Build history of the part. All positions in model axes, mm. Face numbers are marked on the shaded views. A direction names the side the tool comes from. Round coordinates to 2 decimals unless told otherwise and drop trailing zeros. Write each loop counter-clockwise with the first axis right and the second up, starting at its lowest first coordinate (ties: lowest second). Pieces come first, ordered by that corner, then holes. Notation, with made-up numbers: M 4,-32.5 L 58,-32.5 A24 cw 58,-13.5 Z; hole C -39.5,26.25 d6. An arc over 180 degrees is marked long. Write item = value, one per line. Start each with the question number.
Q1. Tool access for the marked faces 4, 5, 6 and 7: list every direction of +Z, -Z, +X, -X, +Y, -Y with a clear straight run to the whole face (end or side of a thin tool).
Q2. Probe L1, parallel to Z at x = 43.5, y = 18; L2, parallel to X at y = 62, z = -44.5; L3, parallel to Y at x = 16.5, z = -11. List the from-to ranges inside material, lowest first.
Q3. Pull direction Z, two halves, no side cores. Call the marked faces 1, 2 and 3: released by +Z, released by -Z, zero draft, split by the parting line, or undercut.
Q4. Drop flat-ended pins along their axis: P1, Ø4, axis at x = 55.5, z = -4.5, coming from the +Y side; P2, Ø6.5, axis at x = 56.34, z = -56.11, coming from the -Y side; P3, Ø2.5, axis at x = -4, y = 41.5, coming from the -Z side; P4, Ø9, axis at x = -5, y = 58.5, coming from the +Z side. Give the stop position or say it passes through.
Q5. Band-saw the part on B-B on z = -13. Write the cut outline in (x, y), plus the area to 3 significant figures.
Q6. Band-saw the part on D-D on x = 40. Write the cut outline in (y, z), plus the area to 3 significant figures.
Q7. Band-saw the part on A-A on y = 16.5. Write the cut outline in (x, z), plus the area to 3 significant figures.
Q8. Band-saw the part on C-C on y = 45. Write the cut outline in (x, z), plus the area to 3 significant figures.
```python
from build123d import *

# Parameters (mm, degrees)
SKETCH1_W            = 62
SKETCH1_H            = 61.770504471
SKETCH1_R            = 4
SKETCH1_R_2          = 27.5
SKETCH1_R_3          = 2
SKETCH1_R_4          = 22.5
BOSS_EXTRUDE6_DEPTH  = 8
SKETCH1_15_W         = 78
SKETCH1_15_H         = 77.770504471
SKETCH1_15_W_2       = 62
SKETCH1_15_H_2       = 61.770504471
BOSS_EXTRUDE9_DEPTH  = 69
SKETCH1_17_R         = 4
CUT_EXTRUDE2_DEPTH   = 56
SKETCH1_18_R         = 4
SKETCH1_18_R_2       = 2
BOSS_EXTRUDE10_DEPTH = 4
FILLET3_R            = 10
CUT_EXTRUDE10_DEPTH  = 8
CUT_EXTRUDE11_DEPTH  = 8
SKETCH6_W            = 21
SKETCH6_H            = 37
CUT_EXTRUDE13_DEPTH  = 10


with BuildPart() as part:
    # Sketch1 → Boss-Extrude6 (new body)
    # profile 1 of 11: a face of its own
    with BuildSketch(Plane(origin=(0, 0, 0), x_dir=(1, 0, 0), z_dir=(0, 1, 0))):
        with Locations((31, 30.885252236)):
            Rectangle(SKETCH1_W, SKETCH1_H)
        with Locations((56.343145751, 56.113650222)):
            Circle(SKETCH1_R, mode=Mode.SUBTRACT)
        with Locations((31, 31)):
            Circle(SKETCH1_R_2, mode=Mode.SUBTRACT)
        with Locations((5.656854249, 56.113650222)):
            Circle(SKETCH1_R, mode=Mode.SUBTRACT)
        with Locations((56.343145751, 5.656854249)):
            Circle(SKETCH1_R, mode=Mode.SUBTRACT)
        with Locations((5.656854249, 5.656854249)):
            Circle(SKETCH1_R, mode=Mode.SUBTRACT)
    # profile 2 of 11: a face of its own
    with BuildSketch(Plane(origin=(0, 0, 0), x_dir=(1, 0, 0), z_dir=(0, 1, 0))):
        with Locations((5.656854249, 5.656854249)):
            Circle(SKETCH1_R)
        with Locations((5.656854249, 5.656854249)):
            Circle(SKETCH1_R_3, mode=Mode.SUBTRACT)
    # profile 3 of 11: a face of its own
    with BuildSketch(Plane(origin=(0, 0, 0), x_dir=(1, 0, 0), z_dir=(0, 1, 0))):
        with Locations((5.656854249, 5.656854249)):
            Circle(SKETCH1_R_3)
    # profile 4 of 11: a face of its own
    with BuildSketch(Plane(origin=(0, 0, 0), x_dir=(1, 0, 0), z_dir=(0, 1, 0))):
        with Locations((56.343145751, 5.656854249)):
            Circle(SKETCH1_R)
        with Locations((56.343145751, 5.656854249)):
            Circle(SKETCH1_R_3, mode=Mode.SUBTRACT)
    # profile 5 of 11: a face of its own
    with BuildSketch(Plane(origin=(0, 0, 0), x_dir=(1, 0, 0), z_dir=(0, 1, 0))):
        with Locations((56.343145751, 5.656854249)):
            Circle(SKETCH1_R_3)
    # profile 6 of 11: a face of its own
    with BuildSketch(Plane(origin=(0, 0, 0), x_dir=(1, 0, 0), z_dir=(0, 1, 0))):
        with Locations((56.343145751, 56.113650222)):
            Circle(SKETCH1_R)
        with Locations((56.343145751, 56.113650222)):
            Circle(SKETCH1_R_3, mode=Mode.SUBTRACT)
    # profile 7 of 11: a face of its own
    with BuildSketch(Plane(origin=(0, 0, 0), x_dir=(1, 0, 0), z_dir=(0, 1, 0))):
        with Locations((56.343145751, 56.113650222)):
            Circle(SKETCH1_R_3)
    # profile 8 of 11: a face of its own
    with BuildSketch(Plane(origin=(0, 0, 0), x_dir=(1, 0, 0), z_dir=(0, 1, 0))):
        with Locations((5.656854249, 56.113650222)):
            Circle(SKETCH1_R)
        with Locations((5.656854249, 56.113650222)):
            Circle(SKETCH1_R_3, mode=Mode.SUBTRACT)
    # profile 9 of 11: a face of its own
    with BuildSketch(Plane(origin=(0, 0, 0), x_dir=(1, 0, 0), z_dir=(0, 1, 0))):
        with Locations((5.656854249, 56.113650222)):
            Circle(SKETCH1_R_3)
    # profile 10 of 11: a face of its own
    with BuildSketch(Plane(origin=(0, 0, 0), x_dir=(1, 0, 0), z_dir=(0, 1, 0))):
        with Locations((31, 31)):
            Circle(SKETCH1_R_2)
        with Locations((31, 31)):
            Circle(SKETCH1_R_4, mode=Mode.SUBTRACT)
    # profile 11 of 11: a face of its own
    with BuildSketch(Plane(origin=(0, 0, 0), x_dir=(1, 0, 0), z_dir=(0, 1, 0))):
        with Locations((31, 31)):
            Circle(SKETCH1_R_4)
    extrude(amount=BOSS_EXTRUDE6_DEPTH)

    # Sketch1_15 → Boss-Extrude9 (add)
    with BuildSketch(Plane(origin=(0, 0, 0), x_dir=(1, 0, 0), z_dir=(0, 1, 0))):
        with Locations((31, 30.885252236)):
            Rectangle(SKETCH1_15_W, SKETCH1_15_H)
        with Locations((31, 30.885252236)):
            Rectangle(SKETCH1_15_W_2, SKETCH1_15_H_2, mode=Mode.SUBTRACT)
    extrude(amount=BOSS_EXTRUDE9_DEPTH)

    # Sketch1_17 → Cut-Extrude2 (cut)
    with BuildSketch(Plane(origin=(0, 0, 0), x_dir=(1, 0, 0), z_dir=(0, 1, 0))):
        with Locations(Location((5.656854249, 56.113650222, 0), (0, 0, 270))):
            Circle(SKETCH1_17_R)
        with Locations(Location((56.343145751, 56.113650222, 0), (0, 0, 90))):
            Circle(SKETCH1_17_R)
        with Locations(Location((56.343145751, 5.656854249, 0), (0, 0, 270))):
            Circle(SKETCH1_17_R)
        with Locations(Location((5.656854249, 5.656854249, 0), (0, 0, 90))):
            Circle(SKETCH1_17_R)
    extrude(amount=CUT_EXTRUDE2_DEPTH, mode=Mode.SUBTRACT)

    # Sketch1_18 → Boss-Extrude10 (add)
    # profile 1 of 4: a face of its own
    with BuildSketch(Plane(origin=(0, 0, 0), x_dir=(1, 0, 0), z_dir=(0, 1, 0))):
        with Locations(Location((5.656854249, 56.113650222, 0), (0, 0, 270))):
            Circle(SKETCH1_18_R)
        with Locations(Location((5.656854249, 56.113650222, 0), (0, 0, 270))):
            Circle(SKETCH1_18_R_2, mode=Mode.SUBTRACT)
    # profile 2 of 4: a face of its own
    with BuildSketch(Plane(origin=(0, 0, 0), x_dir=(1, 0, 0), z_dir=(0, 1, 0))):
        with Locations(Location((56.343145751, 56.113650222, 0), (0, 0, 90))):
            Circle(SKETCH1_18_R)
        with Locations(Location((56.343145751, 56.113650222, 0), (0, 0, 90))):
            Circle(SKETCH1_18_R_2, mode=Mode.SUBTRACT)
    # profile 3 of 4: a face of its own
    with BuildSketch(Plane(origin=(0, 0, 0), x_dir=(1, 0, 0), z_dir=(0, 1, 0))):
        with Locations(Location((56.343145751, 5.656854249, 0), (0, 0, 270))):
            Circle(SKETCH1_18_R)
        with Locations(Location((56.343145751, 5.656854249, 0), (0, 0, 270))):
            Circle(SKETCH1_18_R_2, mode=Mode.SUBTRACT)
    # profile 4 of 4: a face of its own
    with BuildSketch(Plane(origin=(0, 0, 0), x_dir=(1, 0, 0), z_dir=(0, 1, 0))):
        with Locations(Location((5.656854249, 5.656854249, 0), (0, 0, 90))):
            Circle(SKETCH1_18_R)
        with Locations(Location((5.656854249, 5.656854249, 0), (0, 0, 90))):
            Circle(SKETCH1_18_R_2, mode=Mode.SUBTRACT)
    extrude(amount=BOSS_EXTRUDE10_DEPTH)

    # Fillet3
    fillet3_edges = [part.edges().sort_by_distance(p)[0] for p in [
        (-8, 34.5, 8),
        (70, 34.5, 8),
        (70, 34.5, -69.770504471),
        (-8, 34.5, -69.770504471),
    ]]
    fillet(fillet3_edges, radius=FILLET3_R)

    # Sketch3 → Cut-Extrude10 (cut)
    with BuildSketch(Plane(origin=(0, 0, -69.770504471), x_dir=(-1, 0, 0), z_dir=(0, 0, -1))):
        Polygon((-42.5, 69), (-42.5, 64), (-19.5, 65), (-19.5, 69), align=None)
    extrude(amount=-CUT_EXTRUDE10_DEPTH, mode=Mode.SUBTRACT)

    # Sketch9 → Cut-Extrude11 (cut)
    with BuildSketch(Plane.XY.offset(8)):
        Polygon((19.5, 69), (19.5, 64), (42.5, 65), (42.5, 69), align=None)
    extrude(amount=-CUT_EXTRUDE11_DEPTH, mode=Mode.SUBTRACT)

    # Sketch6 → Cut-Extrude13 (cut)
    with BuildSketch(Plane.ZY.offset(8)):
        with Locations((-30.885252236, 50.5)):
            Rectangle(SKETCH6_W, SKETCH6_H)
    extrude(amount=-CUT_EXTRUDE13_DEPTH, mode=Mode.SUBTRACT)


solid = part.part
```
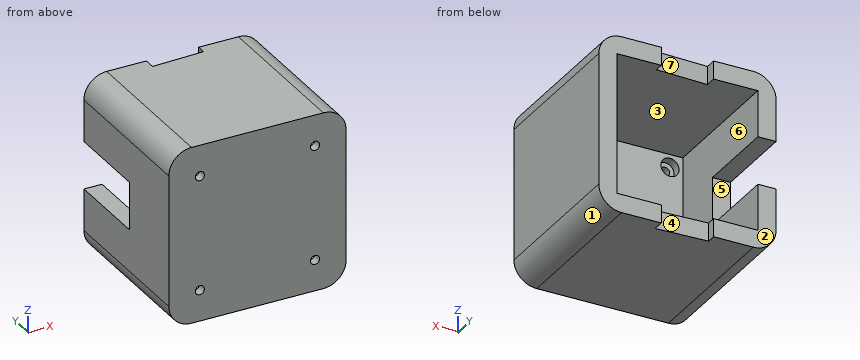
Conclusion:
q1.face_4 = -Z, +Y
q1.face_5 = -X, +Y
q1.face_6 = +Y
q1.face_7 = +Z, +Y
q2.L1 = -69.77 to -61.77, 0 to 8
q2.L2 = -8 to 0, 62 to 70
q2.L3 = 0 to 8
q3.face_1 = released by -Z
q3.face_2 = zero draft
q3.face_3 = undercut
q4.P1 = 4
q4.P2 = 0
q4.P3 = -68.57
q4.P4 = 7.68
q5.outline = M -8,0 L 70,0 L 70,69 L 62,69 L 62,8 L 0,8 L 0,69 L -8,69 Z
q5.area = 1,600 mm^2
q6.outline = M 0,-69.77 L 64.11,-69.77 L 64.11,-61.77 L 8,-61.77 L 8,0 L 64.89,0 L 64.89,8 L 0,8 Z
q6.area = 1,530 mm^2
q7.outline = M -8,-59.77 A10 ccw 2,-69.77 L 60,-69.77 A10 ccw 70,-59.77 L 70,-2 A10 ccw 60,8 L 2,8 A10 ccw -8,-2 Z; hole M 0,-61.77 L 62,-61.77 L 62,0 L 0,0 Z
q7.area = 2,150 mm^2
q8.outline = M -8,-59.77 A10 ccw 2,-69.77 L 60,-69.77 A10 ccw 70,-59.77 L 70,-2 A10 ccw 60,8 L 2,8 A10 ccw -8,-2 L -8,-20.39 L 0,-20.39 L 0,0 L 62,0 L 62,-61.77 L 0,-61.77 L 0,-41.39 L -8,-41.39 Z
q8.area = 1,980 mm^2
